Autodesk Inventor part; units mm, degrees
ref_plane "Work Plane5" through (119.1091, 119.1091, 0) normal (-0.7071, 0.7071, 0) x (-0.7071, -0.7071, 0)
ref_plane "YZ Plane" through (0, 0, 0) normal (1, 0, 0) x (0, 1, 0)
ref_plane "XZ Plane" through (0, 0, 0) normal (0, 1, 0) x (-1, 0, 0)
sketch "Sketch1" plane through (0, 0, 0) normal (0, 0, 1) x (1, 0, 0)
  line L0 (-41.5, 58) -> (41.5, 58)
  line L1 (41.5, 58) -> (41.5, 158)
  line L2 (41.5, 158) -> (-41.5, 158)
  line L3 (-41.5, 158) -> (-41.5, 58)
  line L4 (58, 41.5) -> (158, 41.5)
  line L5 (158, 41.5) -> (158, -41.5)
  line L6 (158, -41.5) -> (58, -41.5)
  line L7 (58, -41.5) -> (58, 41.5)
  line L8 (-131.1952, 0) -> (204.4844, 0) construction
  line L9 (-48, 48) -> (48, 48)
  line L10 (48, 48) -> (48, -48)
  line L11 (48, -48) -> (-48, -48)
  line L12 (-48, -48) -> (-48, 48)
  line L13 (0, 180.9439) -> (0, -136.3054) construction
  point P0 (0, 0)
  point P1 (-48, 0)
  point P2 (0, 48)
  point P3 (0, 58)
  point P4 (58, 0)
  dimension "d0" = 83
  dimension "d1" = 100
  dimension "d2" = 100
  dimension "d3" = 83
  dimension "d5" = 96
  dimension "d6" = 96
  dimension "d7" = 10
  dimension "d8" = 10
sketch "Sketch2" plane through (0, 0, 0) normal (0, 0, 1) x (1, 0, 0)
  line L0 (41.5, 158) -> (-41.5, 158)
  line L1 (41.5, 58) -> (41.5, 158)
  line L2 (-48, 48) -> (48, 48)
  line L3 (48, 48) -> (48, -48)
  line L4 (58, -41.5) -> (58, 41.5)
  line L5 (58, 41.5) -> (158, 41.5)
  line L6 (-41.5, 58) -> (41.5, 58)
  line L7 (158, 41.5) -> (158, -41.5)
  line L8 (48, 48) -> (136.7868, 136.7868) construction
  line L9 (35.5, 78) -> (57.5, 78)
  line L10 (57.5, 78) -> (57.5, 138)
  line L11 (57.5, 138) -> (35.5, 138)
  line L12 (35.5, 138) -> (35.5, 78)
  line L13 (41.5, 108) -> (-41.5, 108) construction
  line L14 (108, 41.5) -> (108, -41.5) construction
  line L15 (41.5, 158) -> (220.1006, 158) construction
  line L16 (158, 41.5) -> (158, 206.0131) construction
  line L17 (115.5736, 158) -> (158, 115.5736) construction
  line L18 (41.5, 138) -> (41.5, 78) construction
  line L19 (51.5, 138) -> (51.5, 78) construction
  line L20 (46.5, 138) -> (46.5, 78) construction
  line L21 (51.5, 158) -> (51.5, 70.6421)
  line L22 (60.0355, 67.1066) -> (133.2513, 140.3223)
  arc A0 (51.5, 158) -> (133.2513, 140.3223) centre (109.2071, 226.9991) ccw
  line L23 (68.9045, 84.4609) -> (84.4609, 68.9045)
  line L24 (84.4609, 68.9045) -> (126.8873, 111.331)
  line L25 (126.8873, 111.331) -> (111.331, 126.8873)
  line L26 (111.331, 126.8873) -> (68.9045, 84.4609)
  line L27 (80.2183, 73.1472) -> (122.6447, 115.5736) construction
  line L28 (105.6741, 90.1177) -> (90.1177, 105.6741) construction
  line L29 (73.1472, 80.2183) -> (115.5736, 122.6447) construction
  line L30 (76.6827, 76.6827) -> (119.1091, 119.1091) construction
  circle A1 centre (73.1472, 84.4609) radius 2.25
  circle A2 centre (111.331, 122.6447) radius 2.25
  circle A3 centre (84.4609, 73.1472) radius 2.25
  circle A4 centre (122.6447, 111.331) radius 2.25
  circle A5 centre (38.5, 135) radius 2.25
  circle A6 centre (38.5, 81) radius 2.25
  circle A7 centre (54.5, 135) radius 2.25
  circle A8 centre (54.5, 81) radius 2.25
  arc A9 (51.5, 70.6421) -> (60.0355, 67.1066) centre (56.5, 70.6421) ccw
  point P0 (0, 0)
  point P1 (158, 158)
  dimension "d23" = 30
  dimension "d25" = 45
  dimension "d30" = 10
  dimension "d37" = 10
  dimension "d38" = 60
  dimension "d39" = 4.5
  dimension "d40" = 3
  dimension "d42" = 4.5
  dimension "d43" = 3
  dimension "d46" = 60
  dimension "d47" = 30
  dimension "d48" = 4.5
  dimension "d49" = 3
  dimension "d50" = 3
  dimension "d51" = 4.5
  dimension "d52" = 3
  dimension "d53" = 3
  dimension "d54" = 5
  dimension "d55" = 25
  dimension "d57" = 3
  dimension "d58" = 3
  dimension "d59" = 3
  dimension "d60" = 3
sketch "Sketch6" plane through (0, 0, 0) normal (0, 0, 1) x (1, 0, 0)
  line L0 (57.5, 138) -> (35.5, 138)
  line L1 (35.5, 138) -> (35.5, 78)
  line L2 (35.5, 78) -> (57.5, 78)
  circle A0 centre (38.5, 81) radius 2.25
  circle A1 centre (38.5, 135) radius 2.25
  circle A2 centre (54.5, 135) radius 2.25
  line L3 (111.331, 126.8873) -> (68.9045, 84.4609)
  circle A3 centre (111.331, 122.6447) radius 2.25
  line L4 (126.8873, 111.331) -> (111.331, 126.8873)
  line L5 (84.4609, 68.9045) -> (126.8873, 111.331)
  line L6 (68.9045, 84.4609) -> (84.4609, 68.9045)
  line L7 (60.0355, 67.1066) -> (133.2513, 140.3223)
  arc A4 (51.5, 70.6421) -> (60.0355, 67.1066) centre (56.5, 70.6421) ccw
  line L8 (51.5, 158) -> (51.5, 70.6421)
  arc A5 (51.5, 158) -> (133.2513, 140.3223) centre (109.2071, 226.9991) ccw
  line L9 (119.1091, 119.1091) -> (76.6827, 76.6827) construction
  circle A6 centre (38.5, 135) radius 2.25
  circle A7 centre (38.5, 81) radius 2.25
  circle A8 centre (54.5, 135) radius 2.25
  circle A9 centre (111.331, 122.6447) radius 2.25
  circle A10 centre (56.5, 70.6421) radius 2.25
  line L10 (57.5, 138) -> (51.5, 138)
  line L11 (35.5, 138) -> (35.5, 78)
  line L12 (57.5, 138) -> (57.5, 83.3339)
  line L13 (111.331, 126.8873) -> (64.3853, 79.9416)
  line L14 (111.331, 126.8873) -> (115.5736, 122.6447)
  line L15 (126.8873, 111.331) -> (84.4609, 68.9045)
  arc A11 (51.5, 70.6421) -> (60.0355, 67.1066) centre (56.5, 70.6421) ccw
  arc A12 (51.5, 70.6421) -> (35.5, 78) centre (33.8506, 53.3381) ccw
  arc A13 (42.2688, 138) -> (51.5, 138) centre (46.8844, 142.3576) ccw
  line L16 (42.2688, 138) -> (35.5, 138)
  arc A14 (115.5736, 122.6447) -> (123.8972, 114.3211) centre (123.1928, 121.9402) ccw
  line L17 (123.8972, 114.3211) -> (126.8873, 111.331)
  arc A15 (57.5, 83.3339) -> (64.3853, 79.9416) centre (61.7783, 83.3339) ccw
  arc A16 (66.0227, 66.0227) -> (60.0355, 67.1066) centre (61.5732, 58.5223) ccw
  line L18 (66.0227, 66.0227) -> (76.6827, 76.6827)
  line L19 (76.6827, 76.6827) -> (84.4609, 68.9045)
  point P0 (0, 0)
  point P1 (69.6117, 76.6827)
  dimension "d99" = 4.5
extrude "Extrusion13" add sketch "Sketch6" along normal blind 0.6 contours L12 A15 L13 L6 L7 A4 L8 L0 | L8 L2 L1 L0 A13 | L8 A12 L2 | L3 L4 L7 L6 | A14 L4 L5 L6 L7 | L7 L6 L18 A16 | A2 | A3 | A10
ref_plane "Work Plane5" through (119.1091, 119.1091, 0) normal (-0.7071, 0.7071, 0) x (-0.7071, -0.7071, 0)
mirror "Mirror3" about plane through (119.1091, 119.1091, 0) normal (-0.7071, 0.7071, 0) of "Extrusion13"
extrude "Extrusion14" cut sketch "Sketch6" along normal blind 0.6 contours A3
mirror "Mirror4" about plane through (119.1091, 119.1091, 0) normal (-0.7071, 0.7071, 0) of "Extrusion14"
sketch "Sketch8" plane through (0, 0, 0.6) normal (0, 0, 1) x (1, 0, 0)
  line L0 (57.5, 138) -> (51.5, 138)
  arc A0 (51.5, 70.6421) -> (60.0355, 67.1066) centre (56.5, 70.6421) ccw
  line L1 (57.5, 138) -> (51.5, 138)
  line L2 (51.5, 138) -> (51.5, 70.6421)
  line L3 (51.5, 70.6421) -> (57.5, 70.6421)
  line L4 (57.5, 70.6421) -> (57.5, 138)
  line L5 (35.5, 138) -> (35.5, 78)
  line L6 (35.5, 138) -> (42.2688, 138)
  line L7 (42.2688, 138) -> (42.2688, 76.5774)
  line L8 (42.2688, 76.5774) -> (35.5, 76.5774)
  line L9 (35.5, 76.5774) -> (35.5, 138)
  arc A1 (51.5, 70.6421) -> (35.5, 78) centre (33.8506, 53.3381) ccw
  arc A2 (42.2688, 131.917) -> (51.5, 131.7579) centre (47.0049, 138.8311) ccw
  line L10 (35.5, 107.2887) -> (57.5, 107.2887) construction
  line L11 (57.5, 83.3339) -> (57.5, 138)
  line L12 (35.5, 110.2887) -> (57.5, 110.2887)
  line L13 (57.5, 110.2887) -> (57.5, 104.2887)
  line L14 (57.5, 104.2887) -> (35.5, 104.2887)
  line L15 (35.5, 104.2887) -> (35.5, 110.2887)
  line L16 (111.331, 126.8873) -> (115.5736, 122.6447)
  line L17 (115.5736, 122.6447) -> (60.0355, 67.1066)
  line L18 (60.0355, 67.1066) -> (55.7929, 71.3492)
  line L19 (55.7929, 71.3492) -> (111.331, 126.8873)
  line L20 (64.3853, 79.9416) -> (111.331, 126.8873)
  line L21 (64.3853, 79.9416) -> (111.331, 126.8873)
  line L22 (87.8581, 103.4145) -> (103.4145, 87.8581) construction
  line L23 (79.9416, 64.3853) -> (126.8873, 111.331)
  line L24 (89.9794, 105.5358) -> (105.5358, 89.9794)
  line L25 (105.5358, 89.9794) -> (101.2931, 85.7368)
  line L26 (101.2931, 85.7368) -> (85.7368, 101.2931)
  line L27 (85.7368, 101.2931) -> (89.9794, 105.5358)
  arc A3 (51.5, 70.6421) -> (60.0355, 67.1066) centre (56.5, 70.6421) ccw
  arc A4 (57.5, 83.3339) -> (64.3853, 79.9416) centre (61.7783, 83.3339) ccw
  arc A5 (57.5, 83.3339) -> (64.3853, 79.9416) centre (61.7783, 83.3339) ccw
  arc A6 (76.6827, 76.6827) -> (69.6117, 76.6827) centre (73.1472, 72.5977) ccw
  line L28 (76.6827, 76.6827) -> (78.804, 78.804)
  arc A7 (78.804, 78.804) -> (73.1472, 80.2183) centre (74.8151, 74.869) ccw
  line L29 (42.2688, 131.917) -> (42.2688, 138)
  line L30 (51.5, 131.7579) -> (51.5, 138)
  line L31 (73.1472, 80.2183) -> (69.6117, 76.6827)
  line L32 (126.8873, 111.331) -> (122.6447, 115.5736)
  arc A8 (117.1923, 117.1923) -> (122.6447, 115.5736) centre (121.9402, 123.1928) ccw
  arc A9 (115.5736, 122.6447) -> (122.6447, 115.5736) centre (121.4114, 121.4114) ccw
  arc A10 (110.6174, 117.6885) -> (113.3377, 113.3377) centre (121.4114, 121.4114) ccw
  arc A11 (115.5736, 122.6447) -> (117.1923, 117.1923) centre (123.1928, 121.9402) ccw
  line L33 (111.331, 126.8873) -> (115.5736, 122.6447)
  line L34 (115.5736, 122.6447) -> (110.6174, 117.6885)
  arc A12 (51.5, 77.7274) -> (35.5, 84.6602) centre (34.6745, 60.8256) ccw
  line L35 (35.5, 85.7368) -> (35.5, 78)
  line L36 (51.5, 78.804) -> (51.5, 70.6421)
  arc A13 (51.5, 70.6421) -> (35.5, 78) centre (33.8506, 53.3381) ccw
  arc A14 (42.2688, 138) -> (51.5, 138) centre (46.8844, 142.3576) ccw
  line L37 (42.2688, 138) -> (35.5, 138)
  arc A15 (42.2688, 138) -> (51.5, 138) centre (46.8844, 142.3576) ccw
  line L38 (117.1923, 117.1923) -> (113.3377, 113.3377)
  arc A16 (68.3773, 68.3773) -> (63.1267, 70.1978) centre (62.8115, 60.8068) ccw
  arc A17 (66.0227, 66.0227) -> (60.0355, 67.1066) centre (61.5732, 58.5223) ccw
  line L39 (68.3773, 68.3773) -> (66.0227, 66.0227)
  line L40 (57.5, 138) -> (57.5, 83.3339)
  line L41 (57.5, 83.3339) -> (57.5, 73.0563)
  line L42 (57.5, 73.0563) -> (64.3853, 79.9416)
  point P0 (0, 0)
  point P1 (35.5, 107.2887)
  dimension "d114" = 6
  dimension "d117" = 3
extrude "Extrusion15" add sketch "Sketch8" along normal blind 0.6 contours L4 L12 L2 L0 | L2 A2 L7 A14 | L4 L14 L2 L12 | L7 L12 L5 L6 | L4 L19 L18 L3 L2 L14 | L2 L14 L7 L12 | A4 L19 L4 | L7 L14 L5 L12 | L19 L26 L17 L18 L3 L4 | L4 L3 L18 L19 | L7 A12 L5 L14 | L19 L24 L17 L26 | L2 A1 L7 A12 | L7 A1 L5 A12 | L18 A0 L3 | L19 L16 L17 L24 | L17 L24 L23 L26 | L17 A16 L39 A17 | A7 L28 A6 L17 | A9 L38 A10 L17 | A11 A9
extrude "Extrusion16" cut sketch "Sketch6" along normal blind 3 contours A0 | A1 | A2 | A3 | A10
mirror "Mirror5" about plane through (119.1091, 119.1091, 0) normal (-0.7071, 0.7071, 0) of "Extrusion15", "Extrusion16"
properties part number "SolarFolds_Sketch"
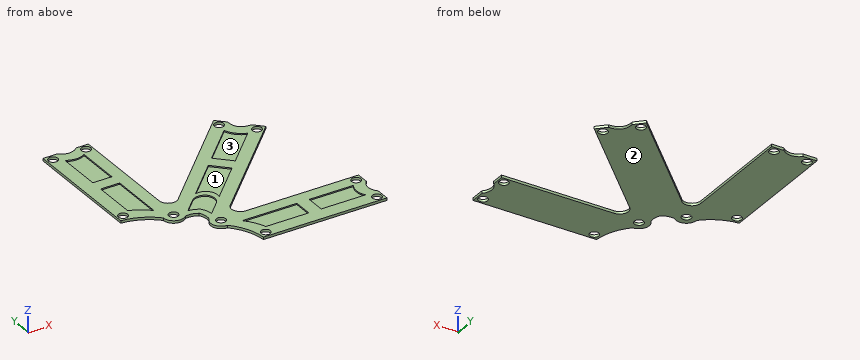
CAD build for the part. Positions are in the model's coordinates, mm. Face numbers are marked on the shaded views. Round coordinates to 2 decimals unless told otherwise and drop trailing zeros. Write each loop counter-clockwise with the first axis right and the second up, starting at its lowest first coordinate (ties: lowest second). Pieces come first, ordered by that corner, then holes. Notation, with made-up numbers: (89, 64.25) - (99, 64.25) arc R32 cw to (99, 91.25) - close; hole circle Ø7 at (26, 74). An arc over 180 degrees is marked (long way). Return JSON: item names as keys, results as strings. Group by question number.
Item 1: Probe probe 1 along Y at (x, z) = (135, 0.2); probe 2 along Y at (x, z) = (113, 0.7). List the from-to ranges inside material, lowest first.
Item 2: Band-saw the part on C-C on z = 0.25. State how many separate pieces and enclosed holes the cut face has, plus the area to 3 significant figures.
Item 3: Mould opens along X. For the marked faces 1, 2 and 3 say: +X half, -X half, draft (parallel to the pull), parting line (faces both ways), or undercut.
Item 4: Band-saw the part on A-A on y = 38.5. List the corners of the cut face in (x, z), plus the area to 3 significant figures.
Item 5: Flat gauge pins, fed straight in: pin 1 Ø0.5 at (y, z) = (45.5, 1) entering from -X; pin 2 Ø0.5 at (y, z) = (96.5, 1) entering from +X; pin 3 Ø0.7 at (y, z) = (47, 1) entering from +X; pin 4 Ø3.5 at (x, y) = (135, 38.5) entering from +Z. Where does each tip first touch, or does it go through?
Resolved:
{
 "1": {"probe 1": "y = 35.5 to 36.25, 40.75 to 52.25, 56.75 to 57.5", "probe 2": "y = 35.5 to 42.27, 51.5 to 57.5, 97.44 to 105.93, 113.69 to 121.14, 124.15 to 125.22"},
 "2": {"separate pieces": "1", "enclosed holes": "10", "area": "4,410 mm²"},
 "3": {"face 1": "undercut", "face 2": "draft", "face 3": "undercut"},
 "4": {"outline": "(77.61, 0) - (78.75, 0) - (78.75, 1.2) - (77.61, 1.2) - close; (83.25, 0) - (132.75, 0) - (132.75, 1.2) - (83.25, 1.2) - close; (137.25, 0) - (138, 0) - (138, 1.2) - (137.25, 1.2) - close", "area": "61.7 mm²"},
 "5": {"pin 1": "stops at x = 75", "pin 2": "stops at x = 112.31", "pin 3": "stops at x = 136.03", "pin 4": "passes through"}
}
